Build history of the part. All positions in model axes, mm. Round coordinates to 2 decimals unless told otherwise and drop trailing zeros. Order: outer loops, then holes, each group sorted by start corner. A loop starts at its lowest first (then second) coordinate and runs counter-clockwise, first axis right, second up. Notation, with made-up numbers: (65.5, 47) -> (93.5, 47) arc R22 cw to (93.5, 57) -> close; hole circle Ø3 at (22.25, 13.5). An arc over 180 degrees is marked (long way). Answer as a JSON object with one key per item and string values.
from build123d import *

# Parameters (mm, degrees)
F0_W           = 55
F0_H           = 70
F1_DEPTH       = 5
F2_D           = 3.3
F2_CSINK_D     = 6.72
F2_CSINK_ANGLE = 90
F3_D           = 2.7
F4_W           = 35
F4_H           = 50
F5_DEPTH       = 5
F6_R           = 6


with BuildPart() as f1:
    # F0 (on Front) → F1 (new body)
    with BuildSketch(Plane.XZ):
        Rectangle(F0_W, F0_H)
    extrude(amount=F1_DEPTH)

    # F2 (through all)
    with Locations(Plane(origin=(0, 0, 0), x_dir=(1, 0, 0), z_dir=(0, 1, 0))):
        with Locations((22.5, -15), (22.5, 30), (-22.5, 30), (-22.5, -15)):
            CounterSinkHole(F2_D / 2, F2_CSINK_D / 2, counter_sink_angle=F2_CSINK_ANGLE)

    # F3 (through all)
    with Locations(Plane(origin=(0, 0, 0), x_dir=(1, 0, 0), z_dir=(0, 1, 0))):
        with Locations((22.5, -30), (-22.5, -30), (-22.5, 15), (22.5, 15)):
            Hole(F3_D / 2)

    # F4 (on face) → F5 (cut, through all)
    with BuildSketch(Plane.XZ.offset(5)):
        Rectangle(F4_W, F4_H)
    extrude(amount=-F5_DEPTH, mode=Mode.SUBTRACT)

    # F6
    f6_edges = [f1.edges().sort_by_distance(p)[0] for p in [
        (-27.5, -2.5, 35),
        (-27.5, -2.5, -35),
        (27.5, -2.5, 35),
        (27.5, -2.5, -35),
        (-17.5, -2.5, -25),
        (17.5, -2.5, 25),
        (17.5, -2.5, -25),
        (-17.5, -2.5, 25),
    ]]
    fillet(f6_edges, radius=F6_R)


solid = f1.part
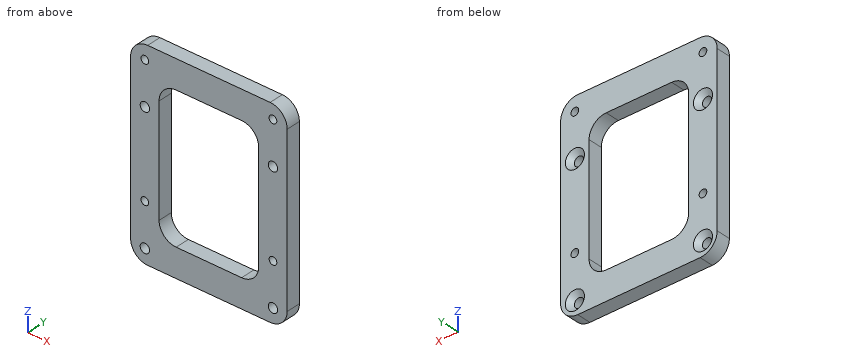
1) Cut at C-C, the plane z = 15. Give the cut face in (x, y).
Checked values:
{"outline": "(-27.5, -5) -> (-24.15, -5) -> (-24.15, -1.71) -> (-25.86, 0) -> (-27.5, 0) -> close; (-20.85, -5) -> (-17.5, -5) -> (-17.5, 0) -> (-19.14, 0) -> (-20.85, -1.71) -> close; (17.5, -5) -> (20.85, -5) -> (20.85, -1.71) -> (19.14, 0) -> (17.5, 0) -> close; (24.15, -5) -> (27.5, -5) -> (27.5, 0) -> (25.86, 0) -> (24.15, -1.71) -> close"}
2) Cut at B-B, the plane y = -3.85. Count the separate pieces of the cut face and the enclosed holes in it, plus the area to 3 significant figures.
Checked values:
{"separate pieces": "1", "enclosed holes": "9", "area": "2,040 mm²"}
3) Flat gauge pin, fed straight in: pin 1 Ø3 at (x, z) = (22.5, 15) entering from -Y. Where does the tip first touch, or does it go through?
Checked values:
{"pin 1": "passes through"}
4) Cut at A-A, the plane x = -1.5. Give the cut face in (y, z).
Checked values:
{"outline": "(-5, -35) -> (0, -35) -> (0, -25) -> (-5, -25) -> close; (-5, 25) -> (0, 25) -> (0, 35) -> (-5, 35) -> close"}
5) Cut at D-D, the plane z = 30. Give the cut face in (x, y).
Checked values:
{"outline": "(-27.42, -5) -> (-23.85, -5) -> (-23.85, 0) -> (-27.42, 0) -> close; (-21.15, -5) -> (21.15, -5) -> (21.15, 0) -> (-21.15, 0) -> close; (23.85, -5) -> (27.42, -5) -> (27.42, 0) -> (23.85, 0) -> close"}
6) Probe L1, parallel to X at y = -4.05, z = 15; L2, parallel to X at y = -3.4, z = -15; L3, parallel to X at y = -4.45, z = 5.5. List the from-to ranges inside material, lowest first. Write a range as from..to.
Checked values:
{"L1": "x = -27.5..-24.15, -20.85..-17.5, 17.5..20.85, 24.15..27.5", "L2": "x = -27.5..-23.85, -21.15..-17.5, 17.5..21.15, 23.85..27.5", "L3": "x = -27.5..-17.5, 17.5..27.5"}
